```python
from build123d import *

# Parameters (mm, degrees)
ESQUISSE1_W                  = 50
ESQUISSE1_H                  = 50
BOSS_EXTRU_1_DEPTH           = 1.6
ESQUISSE2_R                  = 1.75
ENL_V_MAT_EXTRU_1_DEPTH      = 1
ENL_V_MAT_EXTRU_1_DEPTH_BACK = 2.6
ESQUISSE3_W                  = 5
ESQUISSE3_H                  = 20
BOSS_EXTRU_2_DEPTH           = 25


with BuildPart() as part:
    # Esquisse1 → Boss.-Extru.1 (new body)
    with BuildSketch(Plane.XY):
        with Locations((25, 25)):
            Rectangle(ESQUISSE1_W, ESQUISSE1_H)
    extrude(amount=BOSS_EXTRU_1_DEPTH)

    # Esquisse2 → Enlèv. mat.-Extru.1 (cut, two sides)
    with BuildSketch(Plane.XY.offset(1.6)) as enl_v_mat_extru_1_sk:
        with Locations((3, 3)):
            Circle(ESQUISSE2_R)
        with Locations((47, 3)):
            Circle(ESQUISSE2_R)
        with Locations((47, 47)):
            Circle(ESQUISSE2_R)
        with Locations((3, 47)):
            Circle(ESQUISSE2_R)
    extrude(amount=ENL_V_MAT_EXTRU_1_DEPTH, mode=Mode.SUBTRACT)
    extrude(enl_v_mat_extru_1_sk.sketch, amount=-ENL_V_MAT_EXTRU_1_DEPTH_BACK, mode=Mode.SUBTRACT)

    # Esquisse3 → Boss.-Extru.2 (add)
    with BuildSketch(Plane.XY.offset(1.6)):
        with Locations((10.5, 37)):
            Rectangle(ESQUISSE3_W, ESQUISSE3_H)
        with Locations((10.5, 13)):
            Rectangle(ESQUISSE3_W, ESQUISSE3_H)
    extrude(amount=BOSS_EXTRU_2_DEPTH)


solid = part.part
```
Source: CAD feature listing. Evaluate the final solid. Frame: model axes, mm. A direction names the side the tool comes from. Give positions to 0.01 mm unless a question says otherwise; leave off trailing zeros. Write each loop counter-clockwise with the first axis right and the second up, starting at its lowest first coordinate (ties: lowest second). Pieces come first, ordered by that corner, then holes. Notation, with made-up numbers: (86.5, -28.5) - (139.5, -28.5) arc R11 ccw to (139.5, -11.5) - close; hole circle Ø9 at (-17, 26.25). An arc over 180 degrees is marked (long way). One line per item, written item: value. Start each with the question number.
Q1. Material intervals for probe 1 along Y at (x, z) = (3, 1.2); probe 2 along X at (y, z) = (37.5, 7.5); probe 3 along Z at (x, y) = (37, 20.5), sorted ascending. Write a range as from..to.
Q2. First-contact query: pin 1 Ø4 at (x, z) = (5, 5.5) entering from +Y; pin 2 Ø4 at (x, z) = (10, 9.5) entering from -Y; pin 3 Ø10 at (y, z) = (38, 12.5) entering from -X; pin 4 Ø3 at (x, y) = (23, 39) entering from -Z. Flat tips, straight axial feed; report the tip coordinate or a pass-through.
Q3. Section query A-A, the plane x = 3. Return the cut outline in (y, z).
Q4. Section query B-B, the plane z = 25. Return the cut outline in (x, y).
Q5. Section query D-D, the plane x = 35. Return the cut outline in (y, z), then the cut area to 3 significant figures.
Q6. Draft query along X for faces 5 (the face through (0, 25, 1)), 6 (the face through (25, 0, 1)), 7 (the face through (48.617, 2.33, 0.811)). Return one class per face: +X half, -X half, draft (parallel to the pull), parting line (faces both ways), or undercut.
Q7. Set-up query: faces 1 (the face through (10, 47, 14)), 2 (the face through (13, 13, 14)), 3 (the face through (8, 37, 14)), 4 (the face through (10, 3, 14)). Return all of +Z, -Z, +X, -X, +Y, -Y with unobstructed straight access to the full face (end or side cutting, diameter ignored); none if empty.
Q8. Section query C-C, the plane y = 29.5. Return the cut outline in (x, z), then the cut area to 3 significant figures.
Answer:
1. probe 1: y = 0..1.25, 4.75..45.25, 48.75..50
1. probe 2: x = 8..13
1. probe 3: z = 0..1.6
2. pin 1: passes through
2. pin 2: stops at y = 3
2. pin 3: stops at x = 8
2. pin 4: stops at z = 0
3. outline: (0, 0) - (1.25, 0) - (1.25, 1.6) - (0, 1.6) - close; (4.75, 0) - (45.25, 0) - (45.25, 1.6) - (4.75, 1.6) - close; (48.75, 0) - (50, 0) - (50, 1.6) - (48.75, 1.6) - close
4. outline: (8, 3) - (13, 3) - (13, 23) - (8, 23) - close; (8, 27) - (13, 27) - (13, 47) - (8, 47) - close
5. outline: (0, 0) - (50, 0) - (50, 1.6) - (0, 1.6) - close
5. area: 80.0 mm2
6. face 5: -X half
6. face 6: draft
6. face 7: undercut
7. face 1: +Z, +X, -X, +Y
7. face 2: +Z, +X, +Y, -Y
7. face 3: +Z, -X, +Y, -Y
7. face 4: +Z, +X, -X, -Y
8. outline: (0, 0) - (50, 0) - (50, 1.6) - (13, 1.6) - (13, 26.6) - (8, 26.6) - (8, 1.6) - (0, 1.6) - close
8. area: 205 mm2
